For this review, use the dimensioned drawing (mm, ordinates from the lowest corner) and the shaded views. Coordinates: 2 decimals unless noted, no trailing zeros. Order: outer loops, then holes, each group sorted by start corner. A loop starts at its lowest first (then second) coordinate and runs counter-clockwise, first axis right, second up. Notation, with made-up numbers: (66, -6.5) -> (122, -6.5) arc R26 ccw to (122, 23.5) -> close; hole circle Ø5 at (59.5, 57). An arc over 180 degrees is marked (long way). Use one line per item in the form item = value. Start each with the question number.
(1) Wall thickness on line 1 along X through (y, z) = (1.5, 5); line 2 along X through (y, z) = (1.55, 55.85); line 3 along Z through (x, y) = (4.9, 0.4): over which ranges is each line inside the solid? List them lowest first.
(2) Take a section at A-A (y = 0.6). State how many separate pieces and enclosed holes the cut face has, then the cut area to 3 significant figures.
(3) Insertion check: pin 1 Ø1 at (y, z) = (0.5, 24) entering from +X; pin 2 Ø1.3 at (x, z) = (4.9, 106.7) entering from -Y. Each pin has a flat end and moves straight along its axis. Give the tip position at first contact, or say it passes through.
(4) Take a section at B-B (z = 53). State the section outline as (x, y) points.
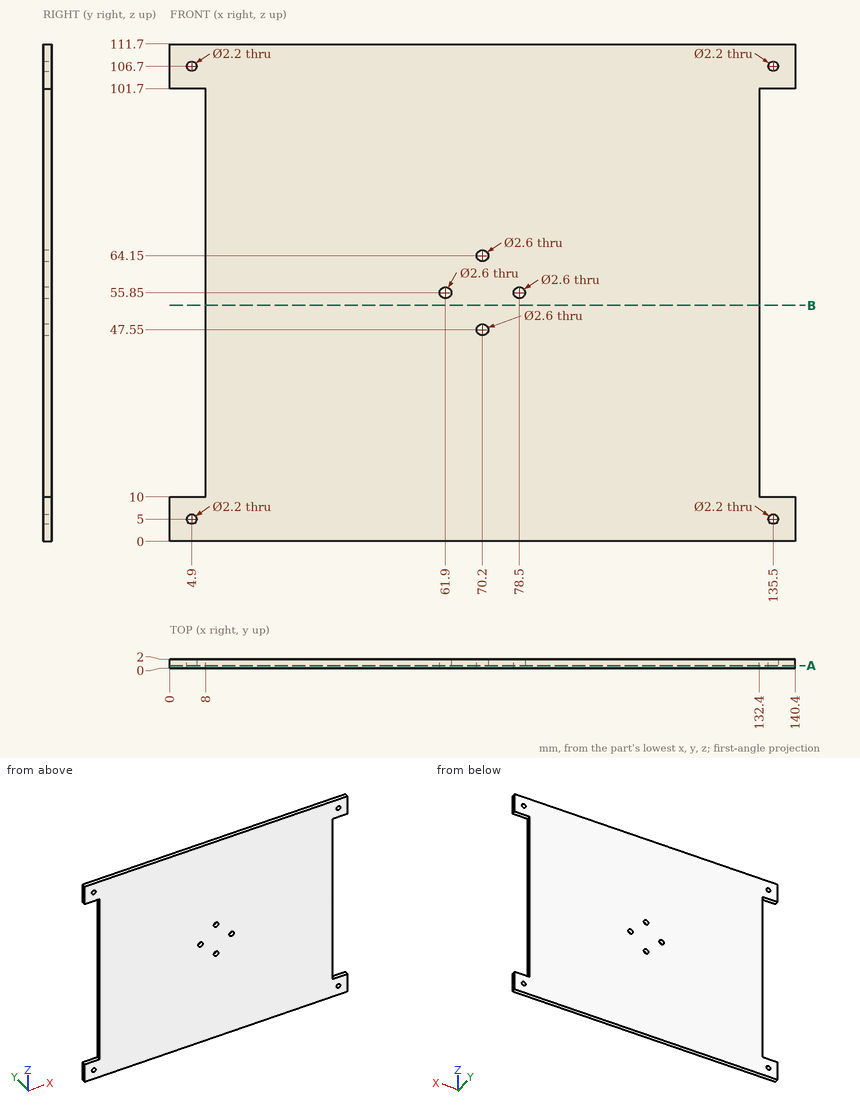
Findings:
q1.line_1 = 0 to 3.8, 6 to 134.4, 136.6 to 140.4
q1.line_2 = 8 to 60.6, 63.2 to 77.2, 79.8 to 132.4
q1.line_3 = 0 to 3.9, 6.1 to 10, 101.7 to 105.6, 107.8 to 111.7
q2.separate_pieces = 1
q2.enclosed_holes = 8
q2.area = 14,200 mm²
q3.pin_1 = 132.4
q3.pin_2 = through
q4.outline = (8, 0) -> (132.4, 0) -> (132.4, 2) -> (8, 2) -> close
